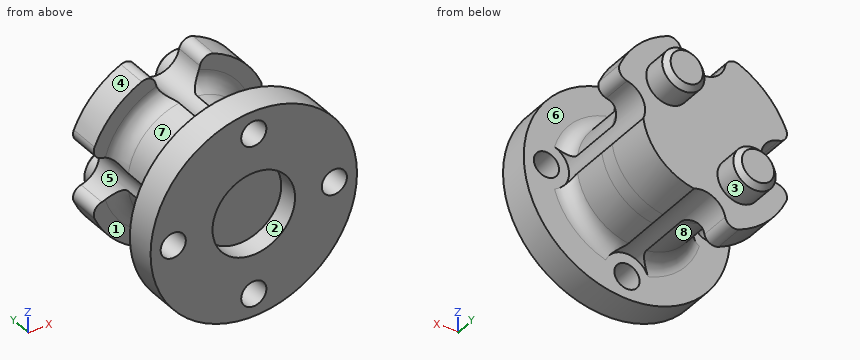
```python
from build123d import *

# Parameters (mm, degrees)
SKETCH3_R           = 1.25
CUT_EXTRUDE1_DEPTH  = 21.152543264
SKETCH4_R           = 2.1
BOSS_EXTRUDE1_DEPTH = 2.8
SKETCH5_R           = 2.25
SKETCH5_R_2         = 1.25
CUT_EXTRUDE2_DEPTH  = 21.014120016
FILLET1_R           = 1.5
CHAMFER1_SIZE       = 0.5
FILLET2_R           = 1
CUT_EXTRUDE3_DEPTH  = 6


with BuildPart() as part:
    # Sketch2 → Revolve2 (revolve)
    with BuildSketch(Plane.XY):
        Polygon((4.1, 2), (4.1, 0), (10.25, 0), (10.25, 3), (6, 3), (6, 11), (9, 11), (9, 14), (0, 14), (0, 2), align=None)
    revolve(axis=Axis((0, 14, 0), (0, -1, 0)))

    # Sketch3 → Cut-Extrude1 (cut, through all)
    with BuildSketch(Plane.XZ):
        with Locations(Location((0, 8, 0), (0, 0, 270))):
            Circle(SKETCH3_R)
        with Locations(Location((8, 0, 0), (0, 0, 270))):
            Circle(SKETCH3_R)
        with Locations(Location((0, -8, 0), (0, 0, 270))):
            Circle(SKETCH3_R)
        with Locations(Location((-8, 0, 0), (0, 0, 270))):
            Circle(SKETCH3_R)
    extrude(amount=-CUT_EXTRUDE1_DEPTH, mode=Mode.SUBTRACT)

    # Sketch4 → Boss-Extrude1 (add)
    with BuildSketch(Plane(origin=(0, 14, 0), x_dir=(1, 0, 0), z_dir=(0, 1, 0))):
        with Locations(Location((-3.535533906, 3.535533906, 0), (0, 0, 270))):
            Circle(SKETCH4_R)
        with Locations(Location((3.535533906, -3.535533906, 0), (0, 0, 270))):
            Circle(SKETCH4_R)
    extrude(amount=BOSS_EXTRUDE1_DEPTH)

    # Sketch5 → Cut-Extrude2 (cut, through all)
    # profile 1 of 4: a face of its own
    with BuildSketch(Plane(origin=(0, 3, 0), x_dir=(1, 0, 0), z_dir=(0, 1, 0))):
        with Locations((0, -8)):
            Circle(SKETCH5_R)
        with Locations(Location((0, -8, 0), (0, 0, 90))):
            Circle(SKETCH5_R_2, mode=Mode.SUBTRACT)
    # profile 2 of 4: a face of its own
    with BuildSketch(Plane(origin=(0, 3, 0), x_dir=(1, 0, 0), z_dir=(0, 1, 0))):
        with Locations((-8, 0)):
            Circle(SKETCH5_R)
        with Locations(Location((-8, 0, 0), (0, 0, 90))):
            Circle(SKETCH5_R_2, mode=Mode.SUBTRACT)
    # profile 3 of 4: a face of its own
    with BuildSketch(Plane(origin=(0, 3, 0), x_dir=(1, 0, 0), z_dir=(0, 1, 0))):
        with Locations((0, 8)):
            Circle(SKETCH5_R)
        with Locations(Location((0, 8, 0), (0, 0, 90))):
            Circle(SKETCH5_R_2, mode=Mode.SUBTRACT)
    # profile 4 of 4: a face of its own
    with BuildSketch(Plane(origin=(0, 3, 0), x_dir=(1, 0, 0), z_dir=(0, 1, 0))):
        with Locations((8, 0)):
            Circle(SKETCH5_R)
        with Locations(Location((8, 0, 0), (0, 0, 90))):
            Circle(SKETCH5_R_2, mode=Mode.SUBTRACT)
    extrude(amount=CUT_EXTRUDE2_DEPTH, mode=Mode.SUBTRACT)

    # Fillet1
    fillet1_edges = [part.edges().sort_by_distance(p)[0] for p in [
        (4.242640687, 11, 4.242640687),
        (4.242640687, 3, 4.242640687),
        (-4.242640687, 11, 4.242640687),
        (-4.242640687, 11, -4.242640687),
        (4.242640687, 11, -4.242640687),
        (-4.242640687, 3, 4.242640687),
        (-4.242640687, 3, -4.242640687),
        (4.242640687, 3, -4.242640687),
    ]]
    fillet(fillet1_edges, radius=FILLET1_R)

    # Chamfer1
    chamfer1_edges = [part.edges().sort_by_distance(p)[0] for p in [
        (-3.535533906, 16.8, -5.635533906),
        (3.535533906, 16.8, 1.435533906),
    ]]
    chamfer(chamfer1_edges, length=CHAMFER1_SIZE)

    # Fillet2
    fillet2_edges = [part.edges().sort_by_distance(p)[0] for p in [
        (-2.122697368, 12.5, 8.74609375),
        (2.122697368, 12.5, 8.74609375),
        (-8.74609375, 12.5, -2.122697368),
        (-8.74609375, 12.5, 2.122697368),
        (2.122697368, 12.5, -8.74609375),
        (-2.122697368, 12.5, -8.74609375),
        (8.74609375, 12.5, 2.122697368),
        (8.74609375, 12.5, -2.122697368),
    ]]
    fillet(fillet2_edges, radius=FILLET2_R)

    # Sketch6 → Cut-Extrude3 (cut)
    with BuildSketch(Plane(origin=(0, 14, 0), x_dir=(1, 0, 0), z_dir=(0, 1, 0))):
        with BuildLine():
            Line((0.89020515, 5.93359375), (0.89020515, 14.456034247))
            Line((0.89020515, 14.456034247), (13.499051384, 10.673985998))
            Line((13.499051384, 10.673985998), (14.247339916, 0.89020515))
            Line((14.247339916, 0.89020515), (5.93359375, 0.89020515))
            ThreePointArc((5.93359375, 0.89020515), (4.242640687, 4.242640687), (0.89020515, 5.93359375))
        make_face()
    extrude(amount=-CUT_EXTRUDE3_DEPTH, mode=Mode.SUBTRACT)


solid = part.part
```
Geometry check sheet. Reference: the model listing, model coordinates, mm. Face numbers are marked on the shaded views. A direction names the side the tool comes from. Round coordinates to 2 decimals unless told otherwise and drop trailing zeros. Order: outer loops, then holes, each group sorted by start corner. A loop starts at its lowest first (then second) coordinate and runs counter-clockwise, first axis right, second up. Notation, with made-up numbers: (15.25, 61.25) - (47.25, 61.25) arc R21 ccw to (47.25, 89.25) - close; hole circle Ø6 at (49, 22.5). An arc over 180 degrees is marked (long way). Use a Markdown table: item, result. Add a question column.
(1) Release check for a two-part mould opening along Z. For the marked faces 1, 2, 3 and 4 record: pulls with the +Z half, pulls with the -Z half, needs draft (parallel to the pull), parting line crosses it, or undercut.
(2) Sectioned sample at A-A, the plane z = 0. Enter the section's corners in (x, y), and give its area (3 significant figures).
(3) Sectioned sample at B-B, the plane y = 9. Enter the section's corners in (x, z), and give its area (3 significant figures).
(4) Tool access check on the marked faces 5, 6, 7 and 8. Record the directions out of +Z, -Z, +X, -X, +Y, -Y that give a thin tool (end or side, any length) a straight path to the whole face; none if there is none.
(5) Sectioned sample at C-C, the plane y = 3.5. Enter the section's corners in (x, z).
(6) Depth check by flat-ended pin: pin 1 (4 mm diameter, centred on x = 1, z = 0, fed in from +Y); pin 2 (2.5 mm diameter, centred on x = -0.5, z = -1.5, fed in from -Y); pin 3 (3 mm diameter, centred on x = 6.5, y = 8.5, fed in from -Z); pin 4 (1.9 mm diameter, centred on x = 5, z = 4.5, fed in from -Y). Enter the tip coordinate at first touch or a pass-through.
(7) Material ranges on line 1 along Y through (x, z) = (4, -8.5); line 2 along Y through (x, z) = (1.25, -2.5); line 3 along X through (y, z) = (2.4, 8), recorded low to high. Write a range as [from, to].
Answers below:
| question | item | result |
|---|---|---|
| 1 | face 1 | needs draft |
| 1 | face 2 | undercut |
| 1 | face 3 | parting line crosses it |
| 1 | face 4 | pulls with the +Z half |
| 2 | outline | (-10.25, 0) - (-9.25, 0) - (-9.25, 3) - (-10.25, 3) - close; (-6.75, 0) - (-4.1, 0) - (-4.1, 2) - (4.1, 2) - (4.1, 0) - (6.75, 0) - (6.75, 3) - (5.75, 3) - (5.75, 14) - (-5.75, 14) - (-5.75, 3) - (-6.75, 3) - close; (9.25, 0) - (10.25, 0) - (10.25, 3) - (9.25, 3) - close |
| 2 | area | 157 mm² |
| 3 | outline | (-5.93, -0.89) arc R6 ccw to (-0.89, -5.93) arc R2.25 cw to (0.89, -5.93) arc R6 ccw to (5.93, -0.89) arc R2.25 cw to (5.93, 0.89) arc R6 ccw to (0.89, 5.93) arc R2.25 cw to (-0.89, 5.93) arc R6 ccw to (-5.93, 0.89) arc R2.25 cw to start |
| 3 | area | 112 mm² |
| 4 | face 5 | -X, +Y |
| 4 | face 6 | none |
| 4 | face 7 | +Z, -X |
| 4 | face 8 | -Z, -X |
| 5 | outline | (-6.23, -1.39) arc R6.38 ccw to (-1.39, -6.23) arc R2.25 cw to (1.39, -6.23) arc R6.38 ccw to (6.23, -1.39) arc R2.25 cw to (6.23, 1.39) arc R6.38 ccw to (1.39, 6.23) arc R2.25 cw to (-1.39, 6.23) arc R6.38 ccw to (-6.23, 1.39) arc R2.25 cw to start |
| 6 | pin 1 | y = 14 |
| 6 | pin 2 | y = 2 |
| 6 | pin 3 | z = -3.32 |
| 6 | pin 4 | y = 0 |
| 7 | line 1 | [0, 3] |
| 7 | line 2 | [2, 14] |
| 7 | line 3 | [-6.41, -1.25], [1.25, 6.41] |
